```python
from build123d import *

# Parameters (mm, degrees)
BOSS_EXTRUDE3_DEPTH       = 50
SKETCH7_W                 = 100
SKETCH7_H                 = 40
CUT_EXTRUDE1_DEPTH        = 11
SKETCH8_R                 = 3.96875
CUT_EXTRUDE2_DEPTH        = 121
CUT_EXTRUDE3_REACH        = 122
SKETCH9_W                 = 20
SKETCH9_H                 = 22
SKETCH10_R                = 3.175
CUT_EXTRUDE4_DEPTH        = 80
SKETCH11_W                = 12.7
SKETCH11_H                = 10
CUT_EXTRUDE5_DEPTH        = 15
F_5_0MM_DOWEL_HOLE1_D     = 5
F_5_0MM_DOWEL_HOLE1_DEPTH = 25
F_5_0MM_DOWEL_HOLE1_TIP   = 1.502151548
SKETCH15_R                = 2.5
CUT_EXTRUDE6_DEPTH        = 15


with BuildPart() as part:
    # Sketch6 → Boss-Extrude3 (new body, symmetric)
    with BuildSketch(Plane.XY):
        Polygon((-60, 22), (-50, 22), (-50, 0), (50, 0), (50, 22), (60, 22), (60, -10), (-60, -10), align=None)
    extrude(amount=BOSS_EXTRUDE3_DEPTH, both=True)

    # Sketch7 → Cut-Extrude1 (cut, through all)
    with BuildSketch(Plane(origin=(0, 0, 0), x_dir=(1, 0, 0), z_dir=(0, 1, 0))):
        with Locations((0, -30)):
            Rectangle(SKETCH7_W, SKETCH7_H)
    extrude(amount=-CUT_EXTRUDE1_DEPTH, mode=Mode.SUBTRACT)

    # Sketch8 → Cut-Extrude2 (cut, through all)
    with BuildSketch(Plane(origin=(60, 0, 0), x_dir=(0, 0, -1), z_dir=(1, 0, 0))):
        with Locations((-30, 10)):
            Circle(SKETCH8_R)
    extrude(amount=-CUT_EXTRUDE2_DEPTH, mode=Mode.SUBTRACT)

    # Sketch9 → Cut-Extrude3 (cut, up to next)
    with BuildSketch(Plane(origin=(60, 0, 0), x_dir=(0, 0, -1), z_dir=(1, 0, 0)), mode=Mode.PRIVATE) as cut_extrude3_sk1:
        with Locations((25, 11)):
            Rectangle(SKETCH9_W, SKETCH9_H)
    cut_extrude3_tool1 = extrude(cut_extrude3_sk1.sketch, amount=-CUT_EXTRUDE3_REACH, mode=Mode.PRIVATE) & part.part
    add(cut_extrude3_tool1.solids().sort_by_distance((60, 11, -25))[0], mode=Mode.SUBTRACT)

    # Sketch10 → Cut-Extrude4 (cut)
    with BuildSketch(Plane.XY.offset(50)):
        with Locations((55, -5)):
            Circle(SKETCH10_R)
    extrude(amount=-CUT_EXTRUDE4_DEPTH, mode=Mode.SUBTRACT)

    # Sketch11 → Cut-Extrude5 (cut)
    with BuildSketch(Plane.XZ.offset(10)):
        with Locations((53.65, 5)):
            Rectangle(SKETCH11_W, SKETCH11_H)
        with Locations((53.65, -12.5)):
            Rectangle(SKETCH11_W, SKETCH11_H)
    extrude(amount=-CUT_EXTRUDE5_DEPTH, mode=Mode.SUBTRACT)

    # Ø5.0mm Dowel Hole1
    with Locations(Plane(origin=(-676.293536786, 42.00000002, -1303.282701689), x_dir=(1, 0, 0), z_dir=(0, 1, 0))):
        with Locations((731.293536786, -1318.853535022), (621.293536786, -1318.853535022), (621.293536786, -1348.282701689), (621.293536786, -1259.995201689), (731.293536786, -1259.995201689), (731.293536786, -1296.570201689), (621.293536786, -1289.424368355), (748.990363778, -1262.26989625)):
            Hole(F_5_0MM_DOWEL_HOLE1_D / 2, depth=F_5_0MM_DOWEL_HOLE1_DEPTH)
            with Locations((0, 0, -(F_5_0MM_DOWEL_HOLE1_DEPTH + F_5_0MM_DOWEL_HOLE1_TIP / 2))):  # 118° drill point
                Cone(0, F_5_0MM_DOWEL_HOLE1_D / 2, F_5_0MM_DOWEL_HOLE1_TIP, mode=Mode.SUBTRACT)

    # Sketch15 → Cut-Extrude6 (cut)
    with BuildSketch(Plane.XZ.offset(10)):
        with Locations((-55, -45)):
            Circle(SKETCH15_R)
        with Locations((-27.5, -45)):
            Circle(SKETCH15_R)
        with Locations((0, -45)):
            Circle(SKETCH15_R)
        with Locations((27.5, -45)):
            Circle(SKETCH15_R)
        with Locations((55, -45)):
            Circle(SKETCH15_R)
    extrude(amount=-CUT_EXTRUDE6_DEPTH, mode=Mode.SUBTRACT)


solid = part.part
```
Input: part model. Units: mm. Frame: model coordinates. A direction names the side the tool comes from. Give positions to 0.01 mm unless a question says otherwise; leave off trailing zeros. Order: outer loops, then holes, each group sorted by start corner. A loop starts at its lowest first (then second) coordinate and runs counter-clockwise, first axis right, second up. Notation, with made-up numbers: (86, 10) -> (128, 10) arc R28 ccw to (128, 46) -> close; hole circle Ø8 at (10, -25.5). An arc over 180 degrees is marked (long way). Write each question's results on one line, items separated by ' | '. Start each with the question number.
Item 1: Cut plane B-B on x = -27.5. Return the cut outline in (y, z), then the cut area to 3 significant figures.
Item 2: Set-up query: faces 5 (the flat face through (55, 13, -15)), 6 (the flat face through (55, -1, 10)), 7 (the cylindrical face through (52.69, 19.47, -42.33)), 8 (the cylindrical face through (57.93, -6.22, -3.7)). Return all of +Z, -Z, +X, -X, +Y, -Y with unobstructed straight access to the full face (end or side cutting, diameter ignored); none if empty.
Item 3: Line query: line 1 (Z direction, x = 55, y = 18.05); line 2 (X direction, y = 20.55, z = 45); line 3 (Z direction, x = -55, y = 20.4). Output: solid intervals per line, ascending.
Item 4: Contact query for flat-ended pins moving along their axis: P1, Ø4.5, axis at x = -55, z = -45, coming from the -Y side; P2, Ø4, axis at x = -11.5, y = -3, coming from the +Z side; P3, Ø3, axis at x = 56, y = -4, coming from the +Z side. Output: stop coordinate, or through.
Item 5: Cut plane A-A on z = 36. Return the cut outline in (x, y) (3 decimals), then the cut area to 3 significant figures.
Item 6: Mould query, pull axis X, two halves, no side actions, for faces 1 (the flat face through (-55, 6, 50)), 2 (the cylindrical face through (-0.54, -5.07, -47.44)), 3 (the conical face through (-54.6, 15.76, -43.12)), 4 (the flat face through (60, 3, -37)). Classes: pulls with the +X half, pulls with the -X half, needs draft (parallel to the pull), parting line crosses it, or undercut.
Item 7: Cut plane C-C on z = -37.5. Return the cut outline in (x, y).
Established:
1) outline: (-10, -50) -> (0, -50) -> (0, -47.5) -> (-10, -47.5) -> close; (-10, -42.5) -> (0, -42.5) -> (0, 10) -> (-10, 10) -> close | area: 550 mm^2
2) face 5: +X, +Y, -Y | face 6: +X, -Y | face 7: +Y | face 8: +Z
3) line 1: -50 to -45.79, -40.79 to -35, -15 to -9.21, -4.21 to 13.07, 18.07 to 50 | line 2: -60 to -57.5, -52.5 to -50, 50 to 60 | line 3: -50 to -45.79, -40.79 to -16.36, -11.36 to 13.07, 18.07 to 42.5, 47.5 to 50
4) P1: y = 5 | P2: z = 10 | P3: z = -30
5) outline: (-60, -10) -> (-50, -10) -> (-50, 22) -> (-60, 22) -> close; (50, -10) -> (60, -10) -> (60, 22) -> (50, 22) -> close; hole circle Ø6.35 at (55, -5) | area: 608 mm^2
6) face 1: needs draft | face 2: undercut | face 3: undercut | face 4: pulls with the +X half
7) outline: (-60, -10) -> (60, -10) -> (60, 22) -> (50, 22) -> (50, 0) -> (-50, 0) -> (-50, 22) -> (-60, 22) -> close
